The listing builds one solid part. Answer for the finished solid, in the listing's coordinates (mm). A direction names the side the tool comes from. Coordinates: 2 decimals unless noted, no trailing zeros. Loops run counter-clockwise (first coordinate to the right, second up) from the corner with the lowest first, then second, coordinate; pieces in that order, holes last. Notation, with made-up numbers: (-19.75, 16) - (36.25, 16) arc R6 ccw to (36.25, 26) - close; hole circle Ø7 at (44.25, 10.25). An arc over 180 degrees is marked (long way). Return JSON: item names as keys, results as strings. Group by question number.
1. Section B-B (z = 5) is taken. Write down the section's boundary in (x, y), and give its area (3 significant figures).
2. Find the intervals of material crossed by line 1 along Z through (x, y) = (6, 1); line 2 along Y through (x, z) = (3.5, 5.75); line 3 along X through (y, z) = (-1, 4.75), in increasing order.
3. Section C-C (x = 4.5) is taken. Write down the section's boundary in (y, z).
4. Section A-A (y = 0) is taken. Write down the section's boundary in (x, z).
5. Section D-D (z = 6.25) is taken. Write down the section's boundary in (x, y).
6. The mould has two halves that part along Z. Classify faces 3 (the face through (7, -2.5, 3)), 4 (the face through (9.5, 0, 4.9)), 5 (the face through (4.283, -0.035, 4.459)): pulls with the +Z half, pulls with the -Z half, needs draft (parallel to the pull), parting line crosses it, or undercut.
7. Which of the six approach directions +Z, -Z, +X, -X, +Y, -Y give full straight-line access (tool end or side, diameter ignored) to faces 1 (the face through (7, 2.5, 3)), 2 (the face through (2, 0, 0))?
8. Each of these flat-tipped pins is pushed along its axis until it touches: P1, Ø2.5, axis at x = 5, y = -0.5, coming from the -Z side; P2, Ø3, axis at x = 7, z = 7, coming from the +Y side; P3, Ø3, axis at x = 7.5, z = 3.5, coming from the -Y side; P4, Ø6, axis at x = 6, z = 5, coming from the -Y side. Where does it stop, or does it pass through?
Autodesk Inventor part; units mm, degrees
ref_plane "YZ Plane" through (0, 0, 0) normal (1, 0, 0) x (0, 1, 0)
ref_plane "XZ Plane" through (0, 0, 0) normal (0, 1, 0) x (-1, 0, 0)
ref_plane "XY Plane" through (0, 0, 0) normal (0, 0, 1) x (1, 0, 0)
sketch "草圖2" plane through (0, 0, 0) normal (0, 0, 1) x (1, 0, 0)
  circle A0 centre (0, 0) radius 1.6
  circle A1 centre (0, 0) radius 4
  dimension "d6" = 3.2
  dimension "d7" = 8
extrude "擠出2" add sketch "草圖2" along normal blind 10
sketch "草圖3" plane through (0, 0, 0) normal (0, 1, 0) x (-1, 0, 0)
  line L0 (0, 2.5) -> (0, 7.5)
  circle A0 centre (-6, 5) radius 1.8
  line L1 (-3, 2.5) -> (-3, 7.5)
  circle A1 centre (-6, 5) radius 3.5
  line L2 (-6, 1.5) -> (0, 1.5)
  line L3 (-6, 8.5) -> (0, 8.5)
  line L4 (0, 8.5) -> (0, 1.5)
  point P0 (0, 0)
  point P1 (-3.8558, -8.4985)
  dimension "d10" = 5
  dimension "d13" = 3.6
  dimension "d16" = 7
extrude "Extrusion4" add sketch "草圖3" along normal mid plane 5
sketch "Sketch5" plane through (0, 0, 8.5) normal (0, 0, 1) x (1, 0, 0)
  circle A0 centre (0, 0) radius 1.6
  dimension "d19" = 3.2
extrude "Extrusion5" cut sketch "Sketch5" along normal through all both and the other way through all
properties part number "避震器上部"
The answers:
{
 "1": {"outline": "(3.12, -2.5) - (4.2, -2.5) - (4.2, 2.5) - (3.12, 2.5) arc R4 ccw (long way) to start; (7.8, -2.5) - (9.5, -2.5) - (9.5, 2.5) - (7.8, 2.5) - close; hole circle Ø3.2 at (0, 0)", "area": "53.1 mm2"},
 "2": {"line 1": "z = 1.5 to 3.2, 6.8 to 8.5", "line 2": "y = -2.5 to 2.5", "line 3": "x = -3.87 to -1.25, 1.25 to 4.22, 7.78 to 9.49"},
 "3": {"outline": "(-2.5, 1.5) - (2.5, 1.5) - (2.5, 4.01) - (-2.5, 4.01) - close; (-2.5, 5.99) - (2.5, 5.99) - (2.5, 8.5) - (-2.5, 8.5) - close"},
 "4": {"outline": "(-4, 0) - (-1.6, 0) - (-1.6, 10) - (-4, 10) - close; (1.6, 0) - (4, 0) - (4, 1.5) - (6, 1.5) arc R3.5 ccw to (6, 8.5) - (4, 8.5) - (4, 10) - (1.6, 10) - close; hole circle Ø3.6 at (6, 5)"},
 "5": {"outline": "(3.12, -2.5) - (4.7, -2.5) - (4.7, 2.5) - (3.12, 2.5) arc R4 ccw (long way) to start; (7.3, -2.5) - (9.27, -2.5) - (9.27, 2.5) - (7.3, 2.5) - close; hole circle Ø3.2 at (0, 0)"},
 "6": {"face 3": "needs draft", "face 4": "parting line crosses it", "face 5": "undercut"},
 "7": {"face 1": "+Z, -Z, +X, +Y", "face 2": "-Z, +X, -X, +Y, -Y"},
 "8": {"P1": "stops at z = 0", "P2": "stops at y = 2.5", "P3": "stops at y = -2.5", "P4": "stops at y = -2.65"}
}
